Geometry check sheet. Reference: the model listing, model coordinates, mm. Face numbers are marked on the shaded views. Give positions to 0.01 mm unless a question says otherwise; leave off trailing zeros. Write each loop counter-clockwise with the first axis right and the second up, starting at its lowest first coordinate (ties: lowest second). Pieces come first, ordered by that corner, then holes. Notation, with made-up numbers: M 25,71 L 53,71 A16 cw 53,93 Z; hole C 61.25,46.25 d2. An arc over 180 degrees is marked long. One line per item, written item: value. Start each with the question number.
1. Scan lines: line 1 (Y direction, x = 0, z = 10.25); line 2 (Y direction, x = -4, z = 3.25); line 3 (Y direction, x = -14, z = 4). Record each from-to range of solid material in increasing order.
2. Cross-section at D-D on x = -10.5. Record the cut outline in (y, z), then the cut area to 3 significant figures.
3. Cross-section at B-B on y = 30.5. Record the cut outline in (x, z).
4. Cross-section at C-C on z = 2.75. Record the cut outline in (x, y).
5. Cross-section at A-A on x = 0. Record the cut outline in (y, z), then the cut area to 3 significant figures.
6. Release check for a two-part mould opening along Y. For the marked faces 1, 2 and 3 record: pulls with the +Y half, pulls with the -Y half, needs draft (parallel to the pull), parting line crosses it, or undercut.
7. Gauge pin test, flat ends, axial feed: pin 1 (10 mm diameter, centred on x = 12.5, y = 31, fed in from -Z); pin 2 (2 mm diameter, centred on x = -9.5, z = 7.5, fed in from +Y); pin 3 (1.5 mm diameter, centred on x = -1, z = 7, fed in from -Y). Record the tip position at first contact, or that the pin passes through.
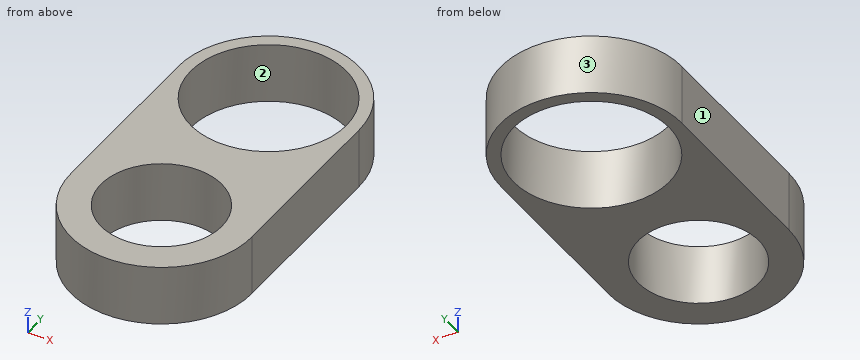
from build123d import *

# Parameters (mm, degrees)
BOSS_EXTRUDE1_DEPTH     = 12.7
CUT_EXTRUDE1_DEPTH      = 62.565534189
CUT_EXTRUDE1_DEPTH_BACK = 62.565534189
SKETCH2_R               = 12.71524
CUT_EXTRUDE2_DEPTH      = 62.565534189
CUT_EXTRUDE2_DEPTH_BACK = 62.565534189
SKETCH3_R               = 16.383


with BuildPart() as part:
    # Sketch1 → Boss-Extrude1 (new body)
    with BuildSketch(Plane.XY):
        with BuildLine():
            Line((-19.05, 0), (-19.05, 38.1))
            ThreePointArc((-19.05, 38.1), (0, 57.15), (19.05, 38.1))
            Line((19.05, 38.1), (19.05, 0))
            ThreePointArc((19.05, 0), (0, -19.05), (-19.05, 0))
        make_face()
    extrude(amount=BOSS_EXTRUDE1_DEPTH)

    # Sketch2 → Cut-Extrude1 (cut, two sides: drawn at the far end of the back side and taken through both)
    with BuildSketch(Plane.XY.offset(12.7).offset(-CUT_EXTRUDE1_DEPTH_BACK)):
        Circle(SKETCH2_R)
    extrude(amount=CUT_EXTRUDE1_DEPTH + CUT_EXTRUDE1_DEPTH_BACK, mode=Mode.SUBTRACT)

    # Sketch3 → Cut-Extrude2 (cut, two sides: drawn at the far end of the back side and taken through both)
    with BuildSketch(Plane.XY.offset(12.7).offset(-CUT_EXTRUDE2_DEPTH_BACK)):
        with Locations((0, 38.1)):
            Circle(SKETCH3_R)
    extrude(amount=CUT_EXTRUDE2_DEPTH + CUT_EXTRUDE2_DEPTH_BACK, mode=Mode.SUBTRACT)


solid = part.part
Report:
1. line 1: y = -19.05 to -12.72, 12.72 to 21.72, 54.48 to 57.15
1. line 2: y = -18.63 to -12.07, 12.07 to 22.21, 53.99 to 56.73
1. line 3: y = -12.92 to 29.59, 46.61 to 51.02
2. outline: M -15.9,0 L -7.17,0 L -7.17,12.7 L -15.9,12.7 Z; M 7.17,0 L 25.52,0 L 25.52,12.7 L 7.17,12.7 Z; M 50.68,0 L 54,0 L 54,12.7 L 50.68,12.7 Z
2. area: 386 mm^2
3. outline: M -19.05,0 L -14.51,0 L -14.51,12.7 L -19.05,12.7 Z; M 14.51,0 L 19.05,0 L 19.05,12.7 L 14.51,12.7 Z
4. outline: M -19.05,0 A19.05 ccw 19.05,0 L 19.05,38.1 A19.05 ccw -19.05,38.1 Z; hole C 0,38.1 d32.77; hole C 0,0 d25.43
5. outline: M -19.05,0 L -12.72,0 L -12.72,12.7 L -19.05,12.7 Z; M 12.72,0 L 21.72,0 L 21.72,12.7 L 12.72,12.7 Z; M 54.48,0 L 57.15,0 L 57.15,12.7 L 54.48,12.7 Z
5. area: 229 mm^2
6. face 1: needs draft
6. face 2: undercut
6. face 3: pulls with the +Y half
7. pin 1: stops at z = 0
7. pin 2: stops at y = 55.15
7. pin 3: stops at y = -19.05
